Input: part model. Units: mm. Frame: model coordinates. A direction names the side the tool comes from. Give positions to 0.01 mm unless a question says otherwise; leave off trailing zeros. Loops run counter-clockwise (first coordinate to the right, second up) from the corner with the lowest first, then second, coordinate; pieces in that order, holes last. Notation, with made-up numbers: (-19, -5) -> (17, -5) arc R24 cw to (17, 32) -> close; hole circle Ø3 at (-12.75, 81). An arc over 180 degrees is marked (long way). One line per question, with ' | ' between items.
from build123d import *

# Parameters (mm, degrees)
BOSS_EXTRUDE1_DEPTH      = 1.5
M3_CLEARANCE_HOLE1_D     = 3.2
M3_CLEARANCE_HOLE1_DEPTH = 3
SKETCH5_R                = 15
CUT_EXTRUDE1_DEPTH       = 1
CUT_EXTRUDE1_DEPTH_BACK  = 4
SKETCH6_R                = 13
BOSS_EXTRUDE2_DEPTH      = 40
M6_CLEARANCE_HOLE1_D     = 6.4
M6_CLEARANCE_HOLE1_DEPTH = 10
CUT_EXTRUDE2_DEPTH       = 40


with BuildPart() as part:
    # Sketch1 → Boss-Extrude1 (new body, symmetric)
    with BuildSketch(Plane(origin=(0, 0, 0), x_dir=(1, 0, 0), z_dir=(0, 1, 0))):
        with BuildLine():
            Line((50, 10), (84, 10))
            ThreePointArc((84, 10), (88.242640687, 8.242640687), (90, 4))
            Line((90, 4), (90, -4))
            ThreePointArc((90, -4), (88.242640687, -8.242640687), (84, -10))
            Line((84, -10), (50, -10))
            ThreePointArc((50, -10), (21.715728753, -21.715728753), (10, -50))
            Line((10, -50), (10, -84))
            ThreePointArc((10, -84), (8.242640687, -88.242640687), (4, -90))
            Line((4, -90), (-4, -90))
            ThreePointArc((-4, -90), (-8.242640687, -88.242640687), (-10, -84))
            Line((-10, -84), (-10, -50))
            ThreePointArc((-10, -50), (-21.715728753, -21.715728753), (-50, -10))
            Line((-50, -10), (-84, -10))
            ThreePointArc((-84, -10), (-88.242640687, -8.242640687), (-90, -4))
            Line((-90, -4), (-90, 4))
            ThreePointArc((-90, 4), (-88.242640687, 8.242640687), (-84, 10))
            Line((-84, 10), (-50, 10))
            ThreePointArc((-50, 10), (-21.715728753, 21.715728753), (-10, 50))
            Line((-10, 50), (-10, 84))
            ThreePointArc((-10, 84), (-8.242640687, 88.242640687), (-4, 90))
            Line((-4, 90), (4, 90))
            ThreePointArc((4, 90), (8.242640687, 88.242640687), (10, 84))
            Line((10, 84), (10, 50))
            ThreePointArc((10, 50), (21.715728753, 21.715728753), (50, 10))
        make_face()
    extrude(amount=BOSS_EXTRUDE1_DEPTH, both=True)

    # M3 Clearance Hole1
    with Locations(Plane(origin=(0, 1.5, 0), x_dir=(1, 0, 0), z_dir=(0, 1, 0))):
        with Locations((-84, 4), (-84, -4), (-4, 84), (4, 84), (84, 4), (84, -4), (4, -84), (-4, -84), (-39, 4), (-39, -4), (39, 4), (39, -4), (4, -39), (-4, -39), (-4, 39), (4, 39)):
            Hole(M3_CLEARANCE_HOLE1_D / 2, depth=M3_CLEARANCE_HOLE1_DEPTH)

    # Sketch5 → Cut-Extrude1 (cut, two sides)
    with BuildSketch(Plane(origin=(0, 1.5, 0), x_dir=(1, 0, 0), z_dir=(0, 1, 0))) as cut_extrude1_sk:
        Circle(SKETCH5_R)
    extrude(amount=CUT_EXTRUDE1_DEPTH, mode=Mode.SUBTRACT)
    extrude(cut_extrude1_sk.sketch, amount=-CUT_EXTRUDE1_DEPTH_BACK, mode=Mode.SUBTRACT)

    # Sketch6 → Boss-Extrude2 (add)
    with BuildSketch(Plane.XZ.offset(1.5)):
        with BuildLine():
            Line((-15.762553167, 8.691485355), (-25.473103505, 18.402035693))
            Line((-25.473103505, 18.402035693), (-18.402035693, 25.473103505))
            Line((-18.402035693, 25.473103505), (-8.691485355, 15.762553167))
            ThreePointArc((-8.691485355, 15.762553167), (12.727922061, 12.727922061), (15.762553167, -8.691485355))
            Line((15.762553167, -8.691485355), (25.473103505, -18.402035693))
            Line((25.473103505, -18.402035693), (18.402035693, -25.473103505))
            Line((18.402035693, -25.473103505), (8.691485355, -15.762553167))
            ThreePointArc((8.691485355, -15.762553167), (-12.727922061, -12.727922061), (-15.762553167, 8.691485355))
        make_face()
        Circle(SKETCH6_R, mode=Mode.SUBTRACT)
    extrude(amount=BOSS_EXTRUDE2_DEPTH)

    # M6 Clearance Hole1
    with Locations(Plane(origin=(3.535533906, 0, 3.535533906), x_dir=(0.707106781, 0, -0.707106781), z_dir=(0.707106781, 0, 0.707106781))):
        with Locations((-24.158012459, -11.5), (-24.158012459, -31.5), (24.158012459, -11.5), (24.158012459, -31.5)):
            Hole(M6_CLEARANCE_HOLE1_D / 2, depth=M6_CLEARANCE_HOLE1_DEPTH)

    # Sketch11 → Cut-Extrude2 (cut)
    with BuildSketch(Plane.XZ.offset(41.5)):
        with BuildLine():
            Line((-21.937569599, 21.937569599), (21.937569599, -21.937569599))
            Line((21.937569599, -21.937569599), (18.402035693, -25.473103505))
            Line((18.402035693, -25.473103505), (8.691485355, -15.762553167))
            ThreePointArc((8.691485355, -15.762553167), (-12.727922061, -12.727922061), (-15.762553167, 8.691485355))
            Line((-15.762553167, 8.691485355), (-25.473103505, 18.402035693))
            Line((-25.473103505, 18.402035693), (-21.937569599, 21.937569599))
        make_face()
    extrude(amount=-CUT_EXTRUDE2_DEPTH, mode=Mode.SUBTRACT)


solid = part.part
1. Pull-direction query (Y, two-part tool) for faces 1 (the cylindrical face through (-14.849, -14.624, 18.335)), 2 (the flat face through (10, -1.5, 9)), 3 (the flat face through (20, -1.5, 19)), 4 (the flat face through (20.55, -21.22, -13.48)); classes: pulls with the +Y half, pulls with the -Y half, needs draft (parallel to the pull), parting line crosses it, or undercut.
Determined:
face 1: undercut | face 2: pulls with the +Y half | face 3: pulls with the -Y half | face 4: needs draft
2. Section query D-D (x = 47.5). Output: boundary loops of the cut face in (y, z), then the cut area to 3 significant figures.
Determined:
outline: (-1.5, -10.08) -> (1.5, -10.08) -> (1.5, 10.08) -> (-1.5, 10.08) -> close | area: 60.5 mm2
3. Pin query (flat end, axial travel): P1, Ø3.5, axis at x = -84, z = -4, coming from the -Y side; P2, Ø3.5, axis at x = -73.5, y = 0.5, coming from the +Z side; P3, Ø2.5, axis at x = 4, z = -84, coming from the -Y side; P4, Ø0.9, axis at x = -72.5, y = 0.5, coming from the -Z side. Return the tip coordinate at first contact, or that it passes through.
Determined:
P1: stops at y = -1.5 | P2: stops at z = 10 | P3: passes through | P4: stops at z = -10
4. Ray query, line 1 along X through (y, z) = (0, -39); line 2 along X through (y, z) = (-0.25, 0); line 3 along X through (y, z) = (0, -84). Return the intervals inside material, ascending. Write a range as from..to.
Determined:
line 1: x = -11.54..-5.6, -2.4..2.4, 5.6..11.54 | line 2: x = -90..-15, 15..90 | line 3: x = -10..-5.6, -2.4..2.4, 5.6..10
5. Section query C-C (z = -43.5). Output: boundary loops of the cut face in (x, y), then the cut area to 3 significant figures.
Determined:
outline: (-10.53, -1.5) -> (10.53, -1.5) -> (10.53, 1.5) -> (-10.53, 1.5) -> close | area: 63.2 mm2
6. Section query A-A (z = 0). Output: boundary loops of the cut face in (x, y), then the cut area to 3 significant figures.
Determined:
outline: (-90, -1.5) -> (-15, -1.5) -> (-15, 1.5) -> (-90, 1.5) -> close; (13, -41.5) -> (18, -41.5) -> (18, -1.5) -> (90, -1.5) -> (90, 1.5) -> (15, 1.5) -> (15, -1.5) -> (13, -1.5) -> close | area: 650 mm2
7. Reachability of faces 5 (the flat face through (-16, -22, 16)), 6 (the flat face through (-13.615, -21.22, 20.686)), 7 (the cylindrical face through (12.496, -21.22, 12.956)), 8 (the cylindrical face through (8.196, 0.021, -88.289)), 9 (the cylindrical face through (-88.289, 0.021, -8.196)) from +Z, -Z, +X, -X, +Y, -Y: full face, straight path, thin tool, end or side. Return the list, or none.
Determined:
face 5: -Z, -X, -Y | face 6: +Z, -Y | face 7: -Y | face 8: -Z, +X, +Y, -Y | face 9: -Z, -X, +Y, -Y
